```python
from build123d import *

# Parameters (mm, degrees)
SKETCH_1_R          = 28
EXTRUDE_1_DEPTH     = 5
EXTRUDE_2_DEPTH     = 20
SKETCH_3_R          = 11
CUT_EXTRUDE_1_DEPTH = 5
EXTRUDE_START       = 5
EXTRUDE_4_DEPTH     = 5


with BuildPart() as part:
    # 草图1 → 凸台-拉伸1 (new body)
    with BuildSketch(Plane.XY):
        Circle(SKETCH_1_R)
    extrude(amount=EXTRUDE_1_DEPTH)

    # 草图2 → 凸台-拉伸2 (add)
    with BuildSketch(Plane(origin=(0, 0, 0), x_dir=(-1, 0, 0), z_dir=(0, 0, -1))):
        with BuildLine():
            Line((-6.498382723, 17.854159795), (-8.892523726, 24.43200814))
            ThreePointArc((-8.892523726, 24.43200814), (0, 26), (8.892523726, 24.43200814))
            Line((8.892523726, 24.43200814), (6.498382723, 17.854159795))
            ThreePointArc((6.498382723, 17.854159795), (0, 19), (-6.498382723, 17.854159795))
        make_face()
        with BuildLine():
            Line((17.854159795, 6.498382723), (24.43200814, 8.892523726))
            ThreePointArc((24.43200814, 8.892523726), (26, 0), (24.43200814, -8.892523726))
            Line((24.43200814, -8.892523726), (17.854159795, -6.498382723))
            ThreePointArc((17.854159795, -6.498382723), (19, 0), (17.854159795, 6.498382723))
        make_face()
        with BuildLine():
            Line((6.498382723, -17.854159795), (8.892523726, -24.43200814))
            ThreePointArc((8.892523726, -24.43200814), (0, -26), (-8.892523726, -24.43200814))
            Line((-8.892523726, -24.43200814), (-6.498382723, -17.854159795))
            ThreePointArc((-6.498382723, -17.854159795), (0, -19), (6.498382723, -17.854159795))
        make_face()
        with BuildLine():
            Line((-17.854159795, -6.498382723), (-24.43200814, -8.892523726))
            ThreePointArc((-24.43200814, -8.892523726), (-26, 0), (-24.43200814, 8.892523726))
            Line((-24.43200814, 8.892523726), (-17.854159795, 6.498382723))
            ThreePointArc((-17.854159795, 6.498382723), (-19, 0), (-17.854159795, -6.498382723))
        make_face()
    extrude(amount=EXTRUDE_2_DEPTH)

    # 草图3 → 切除-拉伸1 (cut)
    with BuildSketch(Plane(origin=(0, 0, 0), x_dir=(-1, 0, 0), z_dir=(0, 0, -1))):
        Circle(SKETCH_3_R)
    extrude(amount=-CUT_EXTRUDE_1_DEPTH, mode=Mode.SUBTRACT)

    # 草图4 → 凸台-拉伸4 (add)
    with BuildSketch(Plane.XY.offset(5).offset(EXTRUDE_START)):
        with BuildLine():
            ThreePointArc((6.880207673, 17.710526316), (0, 26), (-6.880207673, 17.710526316))
            ThreePointArc((-6.880207673, 17.710526316), (0, 19), (6.880207673, 17.710526316))
        make_face()
        with BuildLine():
            ThreePointArc((18.77786954, 2.89682853), (22.516660498, 13), (11.897661868, 14.813697786))
            ThreePointArc((11.897661868, 14.813697786), (16.454482672, 9.5), (18.77786954, 2.89682853))
        make_face()
        with BuildLine():
            ThreePointArc((11.897661868, -14.813697786), (22.516660498, -13), (18.77786954, -2.89682853))
            ThreePointArc((18.77786954, -2.89682853), (16.454482672, -9.5), (11.897661868, -14.813697786))
        make_face()
        with BuildLine():
            ThreePointArc((-6.880207673, -17.710526316), (0, -26), (6.880207673, -17.710526316))
            ThreePointArc((6.880207673, -17.710526316), (0, -19), (-6.880207673, -17.710526316))
        make_face()
        with BuildLine():
            ThreePointArc((-18.77786954, -2.89682853), (-22.516660498, -13), (-11.897661868, -14.813697786))
            ThreePointArc((-11.897661868, -14.813697786), (-16.454482672, -9.5), (-18.77786954, -2.89682853))
        make_face()
        with BuildLine():
            ThreePointArc((-11.897661868, 14.813697786), (-22.516660498, 13), (-18.77786954, 2.89682853))
            ThreePointArc((-18.77786954, 2.89682853), (-16.454482672, 9.5), (-11.897661868, 14.813697786))
        make_face()
    extrude(amount=-EXTRUDE_4_DEPTH)


solid = part.part
```
Build history of the part. All positions in model axes, mm. A direction names the side the tool comes from. Round coordinates to 2 decimals unless told otherwise and drop trailing zeros. Write each loop counter-clockwise with the first axis right and the second up, starting at its lowest first coordinate (ties: lowest second). Pieces come first, ordered by that corner, then holes. Notation, with made-up numbers: (-11.75, 44) - (29.25, 44) arc R33 cw to (29.25, 83) - close; hole circle Ø5 at (65, 1). An arc over 180 degrees is marked (long way). Answer as CSV lines item,"result".
Q1. Pull direction Y, two halves, no side cores. Call faces 1 (the flat face through (-21.189, -7.712, -9.86)), 2 (the flat face through (0, -22, 10)), 3 (the flat face through (-7.712, 21.189, -9.86)): +Y half, -Y half, draft (parallel to the pull), parting line (faces both ways), or undercut.
Report:
face 1,"-Y half"
face 2,"draft"
face 3,"undercut"
Q2. Cut at C-C (y = -4.5). Write the cut outline in (x, z), and give its area (3 significant figures).
Report:
outline,"(-27.64, 0) - (-25.61, 0) - (-25.61, -20) - (-18.46, -20) - (-18.46, 0) - (-10.04, 0) - (-10.04, 5) - (-18.46, 5) - (-18.46, 10) - (-21.35, 10) - (-21.35, 5) - (-27.64, 5) - close; (10.04, 0) - (18.46, 0) - (18.46, -20) - (25.61, -20) - (25.61, 0) - (27.64, 0) - (27.64, 5) - (21.35, 5) - (21.35, 10) - (18.46, 10) - (18.46, 5) - (10.04, 5) - close"
area,"491 mm^2"
Q3. Cut at B-B (z = -5.25). Write the cut outline in (x, y), and give its area (3 significant figures).
Report:
outline,"(-24.43, -8.89) - (-17.85, -6.5) arc R19 cw to (-17.85, 6.5) - (-24.43, 8.89) arc R26 ccw to start; (-8.89, -24.43) arc R26 ccw to (8.89, -24.43) - (6.5, -17.85) arc R19 cw to (-6.5, -17.85) - close; (-8.89, 24.43) - (-6.5, 17.85) arc R19 cw to (6.5, 17.85) - (8.89, 24.43) arc R26 ccw to start; (17.85, -6.5) - (24.43, -8.89) arc R26 ccw to (24.43, 8.89) - (17.85, 6.5) arc R19 cw to start"
area,"440 mm^2"
Q4. Tool access for faces 4 (the cylindrical face through (0, 19, -10)), 5 (the cylindrical face through (0, 19, 8)), 6 (the flat face through (7.68, 21.1, -9.86)), 7 (the flat face through (-7.68, -21.1, -9.86)): list every direction of +Z, -Z, +X, -X, +Y, -Y with a clear straight run to the whole face (end or side of a thin tool).
Report:
face 4,"-Z"
face 5,"+Z"
face 6,"-Z, +X"
face 7,"-Z, -X"
Q5. Cut at A-A (x = 0). Write the cut outline in (y, z).
Report:
outline,"(-28, 0) - (-26, 0) - (-26, -20) - (-19, -20) - (-19, 0) - (-11, 0) - (-11, 5) - (-19, 5) - (-19, 10) - (-26, 10) - (-26, 5) - (-28, 5) - close; (11, 0) - (19, 0) - (19, -20) - (26, -20) - (26, 0) - (28, 0) - (28, 5) - (26, 5) - (26, 10) - (19, 10) - (19, 5) - (11, 5) - close"
Q6. Drill centre lines: probe 1 along Y at (x, z) = (0, 3.65); probe 2 along X at (y, z) = (-2, -11); probe 3 along Y at (x, z) = (5, 3.25). Where is each one in solid material? Low to high. Write a range as [from, to].
Report:
probe 1,"y = [-28, -11], [11, 28]"
probe 2,"x = [-25.92, -18.89], [18.89, 25.92]"
probe 3,"y = [-27.55, -9.8], [9.8, 27.55]"
Q7. Drop flat-ended pins along their axis: pin 1 (6 mm diameter, centred on y = 8, z = 1, fed in from -X); pin 2 (12 mm diameter, centred on y = -12.5, z = -11, fed in from -X); pin 3 (1 mm diameter, centred on x = 4.5, y = 13, fed in from -Z). Give the stop position or say it passes through.
Report:
pin 1,"stops at x = -27.55"
pin 2,"stops at x = -25.17"
pin 3,"stops at z = 0"
Q8. Cut at D-D (x = -21.5). Write the cut outline in (y, z), and give its area (3 significant figures).
Report:
outline,"(-17.94, 0) - (-7.83, 0) - (-7.83, -20) - (7.83, -20) - (7.83, 0) - (17.94, 0) - (17.94, 5) - (14.35, 5) - (14.35, 10) - (4.65, 10) - (4.65, 5) - (-4.65, 5) - (-4.65, 10) - (-14.35, 10) - (-14.35, 5) - (-17.94, 5) - close"
area,"589 mm^2"
